Could you check a few things on this model? Use its own coordinates, in mm. A direction names the side the tool comes from. Coordinates: 2 decimals unless noted, no trailing zeros. Order: outer loops, then holes, each group sorted by start corner. A loop starts at its lowest first (then second) coordinate and runs counter-clockwise, first axis right, second up. Notation, with made-up numbers: (-17, -14) -> (24, -14) arc R19 ccw to (24, 14) -> close; hole circle Ø1 at (1, 73). An arc over 180 degrees is marked (long way). Return JSON: item names as keys, results as strings. Group by question number.
from build123d import *

# Parameters (mm, degrees)
SKETCH1_R           = 7.5
BOSS_EXTRUDE1_DEPTH = 7.5
SKETCH2_R           = 45
BOSS_EXTRUDE2_DEPTH = 70
SKETCH3_W           = 6
SKETCH3_H           = 10
HOLE1_D             = 75


with BuildPart() as part:
    # Sketch1 → Boss-Extrude1 (new body)
    with BuildSketch(Plane(origin=(0, 0, 0), x_dir=(1, 0, 0), z_dir=(0, 1, 0))):
        with BuildLine():
            ThreePointArc((21.819107759, -55.892097264), (51.961524227, -30), (59.313529981, 9.050147025))
            ThreePointArc((59.313529981, 9.050147025), (60.675902532, 15.788685813), (66.066684717, 20.055233762))
            ThreePointArc((66.066684717, 20.055233762), (74.911197427, 43.25), (50.401684275, 47.187810428))
            ThreePointArc((50.401684275, 47.187810428), (44.011354273, 44.652530083), (37.494422222, 46.841950239))
            ThreePointArc((37.494422222, 46.841950239), (0, 60), (-37.494422222, 46.841950239))
            ThreePointArc((-37.494422222, 46.841950239), (-44.011354273, 44.652530083), (-50.401684275, 47.187810428))
            ThreePointArc((-50.401684275, 47.187810428), (-74.911197427, 43.25), (-66.066684717, 20.055233762))
            ThreePointArc((-66.066684717, 20.055233762), (-60.675902532, 15.788685813), (-59.313529981, 9.050147025))
            ThreePointArc((-59.313529981, 9.050147025), (-51.961524227, -30), (-21.819107759, -55.892097264))
            ThreePointArc((-21.819107759, -55.892097264), (-16.664548259, -60.441215897), (-15.665000442, -67.24304419))
            ThreePointArc((-15.665000442, -67.24304419), (0, -86.5), (15.665000442, -67.24304419))
            ThreePointArc((15.665000442, -67.24304419), (16.664548259, -60.441215897), (21.819107759, -55.892097264))
        make_face()
        with Locations(Location((-61.054790967, 35.25, 0), (0, 0, 270))):
            Circle(SKETCH1_R, mode=Mode.SUBTRACT)
        with Locations(Location((61.054790967, 35.25, 0), (0, 0, 270))):
            Circle(SKETCH1_R, mode=Mode.SUBTRACT)
        with Locations(Location((0, -70.5, 0), (0, 0, 270))):
            Circle(SKETCH1_R, mode=Mode.SUBTRACT)
    extrude(amount=BOSS_EXTRUDE1_DEPTH)

    # Sketch2 → Boss-Extrude2 (add)
    with BuildSketch(Plane(origin=(0, 7.5, 0), x_dir=(1, 0, 0), z_dir=(0, 1, 0))):
        with Locations(Location((0, 0, 0), (0, 0, 270))):
            Circle(SKETCH2_R)
    extrude(amount=BOSS_EXTRUDE2_DEPTH)

    # Sketch3 → Cut-Revolve2 (revolve, cut)
    with BuildSketch(Plane.XY, mode=Mode.PRIVATE) as cut_revolve2_sk:
        with Locations((42, 57.5)):
            Rectangle(SKETCH3_W, SKETCH3_H)
        with Locations((42, 32.5)):
            Rectangle(SKETCH3_W, SKETCH3_H)
    revolve(cut_revolve2_sk.sketch.rotate(Axis((0, 0, 0), (0, 1, 0)), 90), axis=Axis((0, 0, 0), (0, 1, 0)), mode=Mode.SUBTRACT)

    # Hole1 (through all)
    with Locations(Plane(origin=(0, 77.5, 0), x_dir=(1, 0, 0), z_dir=(0, 1, 0))):
        with Locations((0, 0)):
            Hole(HOLE1_D / 2)


solid = part.part
Q1. I'm going to push flat-ended pins straight in: pin 1 Ø12 at (x, z) = (0, 70.5) entering from -Y; pin 2 Ø1.5 at (y, z) = (49, -2) entering from -X; pin 3 Ø1.5 at (x, y) = (5, 8) entering from -Z; pin 4 Ø3 at (y, z) = (39.5, -41.5) entering from -X. Where does each tip first touch, or does it pass through?
Q2. I want a section at D-D on y = 59. Please give me the cut outline in (x, z).
Q3. On a 3-axis mill with a long thin cutter (end or side, diameter ignored), from which of +Z, -Z, +X, -X, +Y, -Y can I reach the whole of each face in a straight line? I mean faces 4 (the cylindrical face through (-17.235, 69.895, 41.569)), 5 (the cylindrical face through (16.618, 3.698, 60.528)), 6 (the flat face through (-37, 52.5, -14)). Say none if no direction works.
Q4. I want a section at B-B on z = 0. Please give me the cut outline in (x, y), and give its area (3 significant figures).
Q5. I want a section at C-C on x = 24.5. Please give me the cut outline in (y, z).
Q6. I want a section at A-A on x = 0. State how many separate pieces and enclosed holes the cut face has, and give its area (3 significant figures).
Q7. We'd pull the mould along Y, two halves only. Please class faces 1 (the cylindrical face through (-38.668, 32.57, 5.077)), 2 (the flat face through (34, 77.5, -17)), 3 (the cylindrical face through (-52.24, 3.7, 29.51)): pulls with the +Y half, pulls with the -Y half, needs draft (parallel to the pull), parting line crosses it, or undercut.
Q8. I need wall thicknesses on line 1 along Y through (x, z) = (-19.5, 34.5); line 2 along Z through (x, y) = (1.5, 29.5); line 3 along X through (y, z) = (4.25, 70.5). Which ranges of each line are inside material? Lowest first, please. Write a range as from..to.
Response values:
{
 "1": {"pin 1": "passes through", "pin 2": "stops at x = -44.98", "pin 3": "stops at z = -59.84", "pin 4": "stops at x = -20.62"},
 "2": {"outline": "circle Ø78 at (0, 0); hole circle Ø75 at (0, 0)"},
 "3": {"face 4": "+Y", "face 5": "+X, +Y, -Y", "face 6": "none"},
 "4": {"outline": "(-60, 0) -> (-37.5, 0) -> (-37.5, 77.5) -> (-45, 77.5) -> (-45, 62.5) -> (-39, 62.5) -> (-39, 52.5) -> (-45, 52.5) -> (-45, 37.5) -> (-39, 37.5) -> (-39, 27.5) -> (-45, 27.5) -> (-45, 7.5) -> (-60, 7.5) -> close; (37.5, 0) -> (60, 0) -> (60, 7.5) -> (45, 7.5) -> (45, 27.5) -> (39, 27.5) -> (39, 37.5) -> (45, 37.5) -> (45, 52.5) -> (39, 52.5) -> (39, 62.5) -> (45, 62.5) -> (45, 77.5) -> (37.5, 77.5) -> close", "area": "1,150 mm²"},
 "5": {"outline": "(0, -54.77) -> (7.5, -54.77) -> (7.5, -37.75) -> (27.5, -37.75) -> (27.5, -30.34) -> (37.5, -30.34) -> (37.5, -37.75) -> (52.5, -37.75) -> (52.5, -30.34) -> (62.5, -30.34) -> (62.5, -37.75) -> (77.5, -37.75) -> (77.5, -28.39) -> (0, -28.39) -> close; (0, 28.39) -> (77.5, 28.39) -> (77.5, 37.75) -> (62.5, 37.75) -> (62.5, 30.34) -> (52.5, 30.34) -> (52.5, 37.75) -> (37.5, 37.75) -> (37.5, 30.34) -> (27.5, 30.34) -> (27.5, 37.75) -> (7.5, 37.75) -> (7.5, 54.77) -> (0, 54.77) -> close"},
 "6": {"separate pieces": "3", "enclosed holes": "0", "area": "1,230 mm²"},
 "7": {"face 1": "undercut", "face 2": "pulls with the +Y half", "face 3": "needs draft"},
 "8": {"line 1": "y = 0..27.5, 37.5..52.5, 62.5..77.5", "line 2": "z = -38.97..-37.47, 37.47..38.97", "line 3": "x = -16..-7.5, 7.5..16"}
}
